For this review, take the finished solid that the model builds, in its own axes (mm). A direction names the side the tool comes from. Give positions to 0.01 mm unless a question says otherwise; leave off trailing zeros. Loops run counter-clockwise (first coordinate to the right, second up) from the corner with the lowest first, then second, coordinate; pieces in that order, holes last.
Autodesk Inventor part; units mm, degrees
ref_plane "YZ Plane" through (0, 0, 0) normal (1, 0, 0) x (0, 1, 0)
ref_plane "XZ Plane" through (0, 0, 0) normal (0, 1, 0) x (-1, 0, 0)
ref_plane "XY Plane" through (0, 0, 0) normal (0, 0, 1) x (1, 0, 0)
sketch "Sketch1" plane through (0, 0, 0) normal (1, 0, 0) x (0, 1, 0)
  line L0 (25.646, 15.8058) -> (-25.154, 15.8058)
  line L1 (-25.154, 15.8058) -> (-25.154, -22.2942)
  line L2 (-25.154, -22.2942) -> (25.646, -22.2942)
  line L3 (25.646, -22.2942) -> (25.646, 15.8058)
  point P0 (0, 0)
  dimension "d0" = 50.8
  dimension "d1" = 38.1
extrude "Extrusion1" add sketch "Sketch1" along normal blind 5.08
sketch "Sketch2" plane through (5.08, 0, 0) normal (1, 0, 0) x (0, 0, -1)
  line L0 (-15.8058, 25.646) -> (-15.8058, -25.154)
  line L1 (22.2942, -25.154) -> (22.2942, 25.646)
  line L2 (22.2942, 25.646) -> (-15.8058, 25.646)
  line L3 (-15.8058, -25.154) -> (22.2942, -25.154)
  point P0 (0, 0)
  point P1 (-12.6308, 22.471)
  point P2 (19.1192, 22.471)
  point P3 (19.1192, -21.979)
  point P4 (-12.6308, -21.979)
  dimension "d4" = 3.175
  dimension "d5" = 0
  dimension "d6" = 3.175
  dimension "d7" = 0
  dimension "d8" = 0
  dimension "d9" = 3.175
  dimension "d10" = 0
  dimension "d11" = 3.175
hole "Hole1" at (5.08, 22.471, 12.6308) at (5.08, 22.471, -19.1192) at (5.08, -21.979, -19.1192) at (5.08, -21.979, 12.6308) direction (-1, 0, 0) diameter 2.794 end through all
sketch "Sketch3" plane through (5.08, 0, 0) normal (1, 0, 0) x (0, 0, -1)
  line L0 (-5.6458, 25.646) -> (12.1342, 25.646)
  line L1 (12.1342, 25.646) -> (12.1342, 19.931)
  line L2 (8.9592, 16.756) -> (-2.4708, 16.756)
  line L3 (-5.6458, 19.931) -> (-5.6458, 25.646)
  line L4 (-2.4708, -16.264) -> (8.9592, -16.264)
  line L5 (12.1342, -19.439) -> (12.1342, -25.154)
  line L6 (12.1342, -25.154) -> (-5.6458, -25.154)
  line L7 (-5.6458, -25.154) -> (-5.6458, -19.439)
  line L8 (22.2942, 25.646) -> (-15.8058, 25.646)
  line L9 (-15.8058, -25.154) -> (22.2942, -25.154)
  line L10 (22.2942, -25.154) -> (22.2942, 25.646)
  line L11 (-15.8058, 25.646) -> (-15.8058, -25.154)
  arc A0 (-5.6458, 19.931) -> (-2.4708, 16.756) centre (-2.4708, 19.931) ccw
  arc A1 (8.9592, 16.756) -> (12.1342, 19.931) centre (8.9592, 19.931) ccw
  arc A2 (12.1342, -19.439) -> (8.9592, -16.264) centre (8.9592, -19.439) ccw
  arc A3 (-2.4708, -16.264) -> (-5.6458, -19.439) centre (-2.4708, -19.439) ccw
  point P0 (0, 0)
  point P1 (12.1342, 16.756)
  point P2 (-5.6458, 16.756)
  point P3 (-5.6458, -16.264)
  point P4 (12.1342, -16.264)
  dimension "d19" = 0
  dimension "d20" = 0
  dimension "d21" = 0
  dimension "d22" = 0
  dimension "d23" = 10.16
  dimension "d24" = 10.16
  dimension "d25" = 8.89
  dimension "d26" = 8.89
  dimension "d29" = 3.175
extrude "Extrusion2" cut sketch "Sketch3" against normal blind 20.6375 contours L0 L1 A1 L2 A0 L3 | L7 A3 L4 A2 L5 L6
properties part number "PowerPlugBlockBack"
Item 1: The part is to be moulded in two halves that separate along Y. For faces 1 (the flat face through (3, 0, -22.294)), 2 (the cylindrical face through (2.5, -22.4, 11.3)), 3 (the flat face through (3, 25.646, 11)), say which applies: released by +Y, released by -Y, zero draft, split by the parting line, or undercut.
Answer:
face 1: zero draft
face 2: undercut
face 3: released by +Y
Item 2: Take a section at B-B on x = 1.4. Give the boundary of the cut face in (y, z) (3 decimals).
Answer:
outline: (-25.154, -22.294) - (25.646, -22.294) - (25.646, -12.134) - (19.931, -12.134) arc R3.175 cw to (16.756, -8.959) - (16.756, 2.471) arc R3.175 cw to (19.931, 5.646) - (25.646, 5.646) - (25.646, 15.806) - (-25.154, 15.806) - (-25.154, 5.646) - (-19.439, 5.646) arc R3.175 cw to (-16.264, 2.471) - (-16.264, -8.959) arc R3.175 cw to (-19.439, -12.134) - (-25.154, -12.134) - close; hole circle Ø2.794 at (-21.979, -19.119); hole circle Ø2.794 at (-21.979, 12.631); hole circle Ø2.794 at (22.471, -19.119); hole circle Ø2.794 at (22.471, 12.631)
Item 3: For L1, parallel to Y at x = 3.5, z = -19; L2, parallel to Y at x = 0.35, z = -19.5; L3, parallel to Z at x = 4.6, y = 21, list the stretches that pass through material, from the lowest coordinate up.
Answer:
L1: y = -25.15 to -23.37, -20.59 to 21.08, 23.86 to 25.65
L2: y = -25.15 to -23.32, -20.63 to 21.13, 23.82 to 25.65
L3: z = -22.29 to -12.13, 5.65 to 15.81
Item 4: Take a section at A-A on y = -18. Give the boundary of the cut face in (x, z).
Answer:
outline: (0, -22.29) - (5.08, -22.29) - (5.08, -11.79) - (0, -11.79) - close; (0, 5.3) - (5.08, 5.3) - (5.08, 15.81) - (0, 15.81) - close
Item 5: Take a section at D-D on z = 3.5. Give the boundary of the cut face in (x, y).
Answer:
outline: (0, -16.44) - (5.08, -16.44) - (5.08, 16.93) - (0, 16.93) - close
Item 6: Take a section at C-C on z = -7.5. Give the boundary of the cut face in (x, y).
Answer:
outline: (0, -16.26) - (5.08, -16.26) - (5.08, 16.76) - (0, 16.76) - close
Item 7: Clearance check with flat-ended pins moving along their axes: pin 1 Ø2.5 at (x, z) = (2.5, -5) entering from -Y; pin 2 Ø3 at (x, z) = (1.5, -8.5) entering from +Y. State where each tip first meets the part, or that it passes through.
Answer:
pin 1: stops at y = -16.26
pin 2: stops at y = 16.93
Item 8: Tool access review of faces 4 (the cylindrical face through (2.58, 17.71, 4.74)), 5 (the flat face through (3, -22, -12.134)), 6 (the cylindrical face through (2.504, 21.086, -18.937)): name each direction out of +Z, -Z, +X, -X, +Y, -Y from which nothing blocks a thin tool from reaching the whole face with its end or side.
Answer:
face 4: +X, -X, +Y
face 5: +X, -X, -Y
face 6: +X, -X
